The listing builds one solid part. Answer for the finished solid, in the listing's coordinates (mm). A direction names the side the tool comes from. Give positions to 0.01 mm unless a question says otherwise; leave off trailing zeros. Write each loop counter-clockwise with the first axis right and the second up, starting at its lowest first coordinate (ties: lowest second). Pieces come first, ordered by that corner, then holes. Notation, with made-up numbers: M 57,2.5 L 66,2.5 A22 cw 66,26.5 Z; hole C 56,-12.5 d2. An arc over 180 degrees is marked long. Return JSON: item names as keys, results as strings.
from build123d import *

# Parameters (mm, degrees)
SKETCH1_W           = 80
SKETCH1_H           = 25
BOSS_EXTRUDE1_DEPTH = 5
BOSS_EXTRUDE2_DEPTH = 80
CUT_EXTRUDE1_DEPTH  = 19


with BuildPart() as part:
    # Sketch1 → Boss-Extrude1 (new body)
    with BuildSketch(Plane(origin=(0, 0, 0), x_dir=(1, 0, 0), z_dir=(0, 1, 0))):
        with Locations((40, 12.5)):
            Rectangle(SKETCH1_W, SKETCH1_H)
    extrude(amount=BOSS_EXTRUDE1_DEPTH)

    # Sketch2 → Boss-Extrude2 (add)
    with BuildSketch(Plane.ZY):
        Polygon((-25, 5), (-25, 24), (13, 24), (13, 19), (11, 19), (11, 22), (-23, 22), (-23, 5), align=None)
    extrude(amount=-BOSS_EXTRUDE2_DEPTH)

    # Sketch3 → Cut-Extrude1 (cut)
    with BuildSketch(Plane(origin=(0, 24, 0), x_dir=(1, 0, 0), z_dir=(0, 1, 0))):
        Polygon((59.190693398, 25), (49.569343824, 2.768409055), (29.769781604, 2.768409055), (20.148432029, 25), align=None)
    extrude(amount=-CUT_EXTRUDE1_DEPTH, mode=Mode.SUBTRACT)


solid = part.part
Item 1: Determine the mould class of faces 1 (the flat face through (39, 20, 11)), 2 (the flat face through (69, 14, -23)), 3 (the flat face through (39, 0, -13)) for opening direction Y: +Y half, -Y half, draft (parallel to the pull), parting line (faces both ways), or undercut.
Geometry results:
{"face 1": "draft", "face 2": "undercut", "face 3": "-Y half"}
Item 2: A cutting plane is placed at D-D, the plane z = 2. Write down the section's boundary in (x, y), plus the area to 3 significant figures.
Geometry results:
{"outline": "M 0,22 L 80,22 L 80,24 L 0,24 Z", "area": "160 mm2"}
Item 3: Find the intervals of material crossed by line 1 (Y direction, x = 65.5, z = -6.5); line 2 (Z direction, x = 75.5, y = 8.5); line 3 (Z direction, x = 68.5, y = 19.5), in increasing order.
Geometry results:
{"line 1": "y = 0 to 5, 22 to 24", "line 2": "z = -25 to -23", "line 3": "z = -25 to -23, 11 to 13"}
Item 4: A cutting plane is placed at C-C, the plane x = 73. Write down the section's boundary in (y, z).
Geometry results:
{"outline": "M 0,-25 L 24,-25 L 24,13 L 19,13 L 19,11 L 22,11 L 22,-23 L 5,-23 L 5,0 L 0,0 Z"}
Item 5: Given pin 1 Ø0.9 at (x, y) = (50, 20) entering from -Z; pin 2 Ø5.5 at (x, y) = (46, 2.5) entering from +Z; pin 3 Ø1.6 at (x, y) = (40, 23) entering from -Z, each flat-ended and moving along its own axis, determine where each tip first touches the part or whether it passes through.
Geometry results:
{"pin 1": "stops at z = 11", "pin 2": "stops at z = 0", "pin 3": "stops at z = -2.77"}
Item 6: Which of the six approach directions +Z, -Z, +X, -X, +Y, -Y give full straight-line access (tool end or side, diameter ignored) to faces 4 (the flat face through (40, 23, -2.768)), 5 (the flat face through (0, 4, -12)), 6 (the flat face through (39, 19, 12)), 7 (the flat face through (39, 22, -2))?
Geometry results:
{"face 4": "-Z, +Y", "face 5": "+Z, -Z, -X, +Y, -Y", "face 6": "+Z, +X, -X, -Y", "face 7": "+X, -X"}
Item 7: A cutting plane is placed at A-A, the plane y = 14.75. Write down the section's boundary in (x, z).
Geometry results:
{"outline": "M 0,-25 L 20.15,-25 L 21.01,-23 L 0,-23 Z; M 58.33,-23 L 59.19,-25 L 80,-25 L 80,-23 Z"}
Item 8: A cutting plane is placed at B-B, the plane z = -8.5. Write down the section's boundary in (x, y).
Geometry results:
{"outline": "M 0,0 L 80,0 L 80,5 L 0,5 Z; M 0,22 L 27.29,22 L 27.29,24 L 0,24 Z; M 52.05,22 L 80,22 L 80,24 L 52.05,24 Z"}
